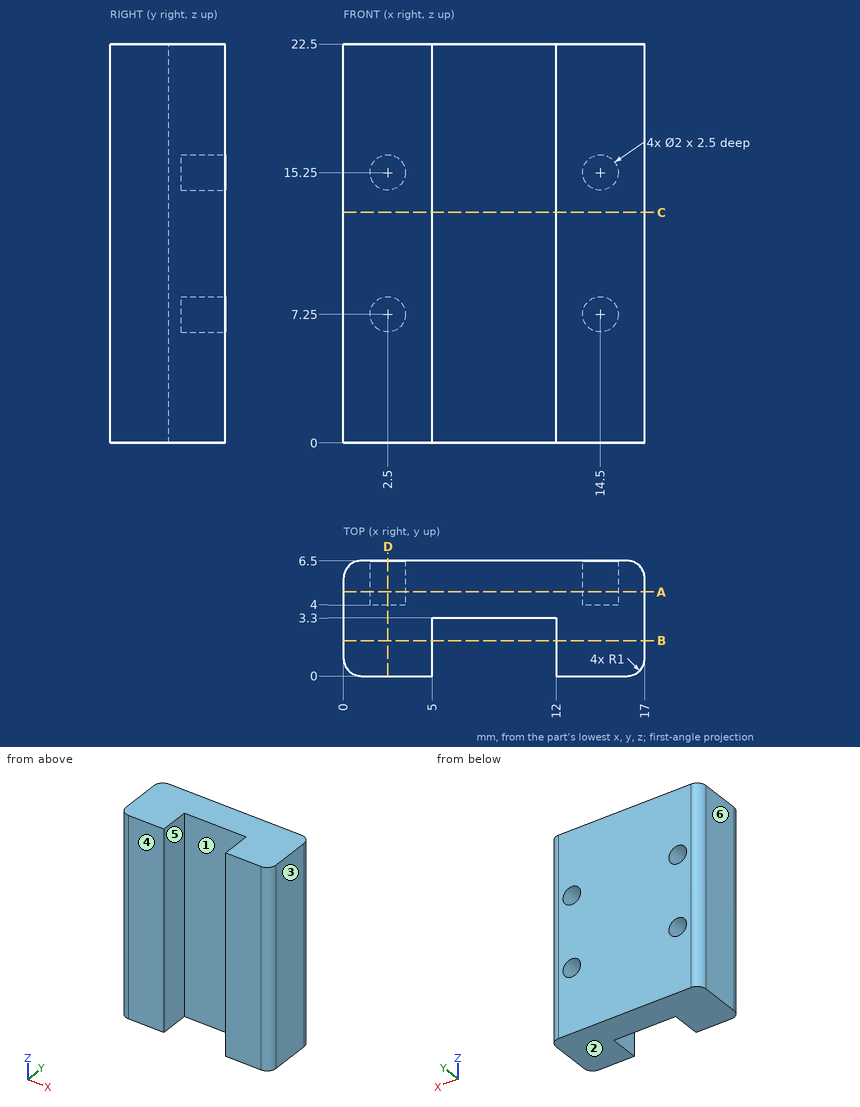
Verification items for this drawing (mm, ordinates from the low corner). A direction names the side the tool comes from. Coordinates: 2 decimals unless noted, no trailing zeros. Write each loop counter-clockwise with the first axis right and the second up, starting at its lowest first coordinate (ties: lowest second). Pieces come first, ordered by that corner, then holes. Notation, with made-up numbers: (10, 49) -> (62, 49) arc R25 ccw to (62, 88) -> close; hole circle Ø4 at (-10.5, 41). An arc over 180 degrees is marked (long way). One line per item, written item: value. Start each with the question number.
Q1. Mould release check, pull along X, two halves, no side actions. Record for the marked faces 3, 4, 5 and 6: pulls with the +X half, pulls with the -X half, needs draft (parallel to the pull), parting line crosses it, or undercut.
Q2. Thickness scan on L1, parallel to Z at x = 14.5, y = 5.7; L2, parallel to X at y = 5, z = 15.25; L3, parallel to X at y = 2.5, z = 9.5. Record the ranges inside material, lowest first. Write a range as from..to.
Q3. Cross-section at A-A on y = 4.75. Enter the section's corners in (x, z), and give its area (3 significant figures).
Q4. Access from +Z, -Z, +X, -X, +Y, -Y to the whole of each face (thin tool, end or side, straight path). Record for the marked faces 1 and 2.
Q5. Cross-section at C-C on z = 13. Enter the section's corners in (x, y).
Q6. Cross-section at D-D on x = 2.5. Enter the section's corners in (y, z), and give its area (3 significant figures).
Q7. Go/stop test with flat-tipped pins: P1, Ø1.6, axis at y = 2.5, z = 10.5, coming from the -X side; P2, Ø0.6, axis at x = 2.5, z = 15, coming from the +Y side. Record where each tip stops, or that it passes through.
Q8. Cross-section at B-B on y = 2. Enter the section's corners in (x, z).
Checked values:
1. face 3: pulls with the +X half
1. face 4: needs draft
1. face 5: undercut
1. face 6: pulls with the -X half
2. L1: z = 0..6.25, 8.25..14.25, 16.25..22.5
2. L2: x = 0..1.5, 3.5..13.5, 15.5..17
2. L3: x = 0..5, 12..17
3. outline: (0, 0) -> (17, 0) -> (17, 22.5) -> (0, 22.5) -> close; hole circle Ø2 at (2.5, 7.25); hole circle Ø2 at (2.5, 15.25); hole circle Ø2 at (14.5, 7.25); hole circle Ø2 at (14.5, 15.25)
3. area: 370 mm²
4. face 1: +Z, -Z, -Y
4. face 2: -Z, +X, -X, +Y, -Y
5. outline: (0, 1) arc R1 ccw to (1, 0) -> (5, 0) -> (5, 3.3) -> (12, 3.3) -> (12, 0) -> (16, 0) arc R1 ccw to (17, 1) -> (17, 5.5) arc R1 ccw to (16, 6.5) -> (1, 6.5) arc R1 ccw to (0, 5.5) -> close
6. outline: (0, 0) -> (6.5, 0) -> (6.5, 6.25) -> (4, 6.25) -> (4, 8.25) -> (6.5, 8.25) -> (6.5, 14.25) -> (4, 14.25) -> (4, 16.25) -> (6.5, 16.25) -> (6.5, 22.5) -> (0, 22.5) -> close
6. area: 136 mm²
7. P1: stops at x = 0
7. P2: stops at y = 4
8. outline: (0, 0) -> (5, 0) -> (5, 22.5) -> (0, 22.5) -> close; (12, 0) -> (17, 0) -> (17, 22.5) -> (12, 22.5) -> close
